Input: part model. Units: mm. Frame: model coordinates. Face numbers are marked on the shaded views. A direction names the side the tool comes from. Round coordinates to 2 decimals unless told otherwise and drop trailing zeros. Order: outer loops, then holes, each group sorted by start corner. A loop starts at its lowest first (then second) coordinate and runs counter-clockwise, first axis right, second up. Notation, with made-up numbers: (0.5, 73.5) -> (10.5, 73.5) arc R8 cw to (10.5, 87.5) -> close; hole circle Ø9 at (84.25, -28). An arc over 180 degrees is marked (long way). Use a Markdown table: item, result.
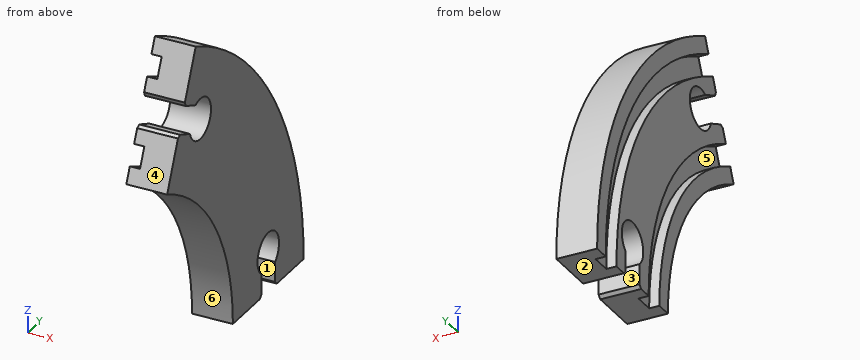
from build123d import *

# Parameters (mm, degrees)
F4_DEPTH = 12.7
F5_SIZE  = 1.016


with BuildPart() as f2:
    # F2: sweep along a path in F1
    with BuildLine(Plane.YZ) as f2_path:
        ThreePointArc((0, 0), (-13.9895526568, 47.0829736144), (-51.4187773904, 78.8881166537))
    # F0 (on Top) → F2 (sweep)
    with BuildSketch(Plane.XY):
        Polygon((-2.9826171882, -15.875), (-2.9826171882, -20.955), (9.7173828118, -20.955), (9.7173828118, 20.955), (-2.9826171882, 20.955), (-2.9826171882, 15.875), (0.1923828118, 15.875), (0.1923828118, 9.525), (-2.9826171882, 9.525), (-2.9826171882, -9.525), (0.1923828118, -9.525), (0.1923828118, -15.875), align=None)
    sweep(path=f2_path.line)

    # F3 (on face) → F4 (cut, through all)
    with BuildSketch(Plane.YZ.offset(9.7173828118)):
        with BuildLine():
            Line((-4.064, 7.3128193311), (-4.064, 0))
            Line((-4.064, 0), (4.064, 0))
            Line((4.064, 0), (4.064, 7.3128193311))
            ThreePointArc((4.064, 7.3128193311), (0, 18.542), (-4.064, 7.3128193311))
        make_face()
        with BuildLine():
            Line((-43.0877289811, 79.6543117793), (-49.7782573242, 82.6062868909))
            Line((-49.7782573242, 82.6062868909), (-53.0592974567, 75.1699464166))
            Line((-53.0592974567, 75.1699464166), (-46.3687691136, 72.217971305))
            ThreePointArc((-46.3687691136, 72.217971305), (-34.4546256835, 71.4032438515), (-43.0877289811, 79.6543117793))
        make_face()
    extrude(amount=-F4_DEPTH, mode=Mode.SUBTRACT)

    # F5
    f5_edges = [f2.edges().sort_by_distance(p)[0] for p in [
        (3.367383, -53.059297, 75.169946),
        (3.367383, -49.778257, 82.606287),
        (3.367383, 4.064, 0),
        (3.367383, -4.064, 0),
    ]]
    chamfer(f5_edges, length=F5_SIZE)


solid = f2.part
1) Pull-direction query (Y, two-part tool) for the marked faces 1, 2, 3 and 4; classes: +Y half, -Y half, draft (parallel to the pull), parting line (faces both ways), or undercut.
Results found:
| item | result |
|---|---|
| face 1 | undercut |
| face 2 | draft |
| face 3 | undercut |
| face 4 | -Y half |
2) Cut plane C-C on y = 0. Return loops of the section in (x, z).
Results found:
| item | result |
|---|---|
| outline | (-2.98, 18.54) -> (9.72, 18.54) -> (9.72, 63.66) -> (-2.98, 63.66) -> (-2.98, 54.68) -> (0.19, 54.68) -> (0.19, 41.63) -> (-2.98, 41.63) -> close |
3) Line query: L1, parallel to Y at x = -0.75, z = 18; L2, parallel to Y at x = -1.5, z = 40; L3, parallel to Y at x = -0.25, z = 69.5. Output: solid intervals per line, ascending. Write a range as [from, to].
Results found:
| item | result |
|---|---|
| L1 | y = [-23.49, -18.22], [-11.67, -2.57], [2.57, 7.82], [14.28, 19.43] |
| L2 | y = [-34.65, -28.35], [-20.78, 0.77], [7.71, 13.21] |
| L3 | y = [-53.78, -44.78], [-35.75, -20.36], [-11.43, -4.63] |
4) Set-up query: the marked faces 5 and 6. Return all of +Z, -Z, +X, -X, +Y, -Y with unobstructed straight access to the full face (end or side cutting, diameter ignored); none if empty.
Results found:
| item | result |
|---|---|
| face 5 | -X |
| face 6 | -Z, +X, -X, -Y |
5) Cut plane A-A on x = 6.5. Return loops of the section in (y, z) (3 decimals), and give its area (3 significant figures).
Results found:
| item | result |
|---|---|
| outline | (-59.878, 59.716) arc R65.271 cw to (-20.955, 0) -> (-5.08, 0) -> (-4.064, 1.016) -> (-4.064, 7.313) arc R6.35 cw (long way) to (4.064, 7.313) -> (4.064, 1.016) -> (5.08, 0) -> (20.955, 0) arc R107.181 ccw to (-42.96, 98.06) -> (-49.368, 83.536) -> (-48.849, 82.196) -> (-43.088, 79.654) arc R6.35 cw (long way) to (-46.369, 72.218) -> (-52.13, 74.76) -> (-53.469, 74.24) -> close |
| area | 3,820 mm² |
6) Pin query (flat end, axial travel): pin 1 Ø4 at (x, y) = (3.5, 10.5) entering from +Z; pin 2 Ø4 at (x, y) = (1, 11.5) entering from +Z; pin 3 Ø5 at (x, z) = (7.5, 69) entering from -Y; pin 4 Ø11.5 at (y, z) = (0, 12.192) entering from +X. Return the tip coordinate at first contact, or that it passes through.
Results found:
| item | result |
|---|---|
| pin 1 | stops at z = 50.15 |
| pin 2 | stops at z = 48.21 |
| pin 3 | stops at y = -56.88 |
| pin 4 | passes through |
7) Cut plane D-D on y = -26.5. Return loops of the section in (x, z), and give its area (3 significant figures).
Results found:
| item | result |
|---|---|
| outline | (-2.98, 26.33) -> (9.72, 26.33) -> (9.72, 89) -> (-2.98, 89) -> (-2.98, 82.81) -> (0.19, 82.81) -> (0.19, 74.84) -> (-2.98, 74.84) -> (-2.98, 48.12) -> (0.19, 48.12) -> (0.19, 37.18) -> (-2.98, 37.18) -> close |
| area | 736 mm² |
8) Cut plane B-B on z = 14.5. Return loops of the section in (x, y), and give its area (3 significant figures).
Results found:
| item | result |
|---|---|
| outline | (-2.98, -22.59) -> (9.72, -22.59) -> (9.72, -5.92) -> (-2.98, -5.92) -> (-2.98, -10.91) -> (0.19, -10.91) -> (0.19, -17.39) -> (-2.98, -17.39) -> close; (-2.98, 5.92) -> (9.72, 5.92) -> (9.72, 19.97) -> (-2.98, 19.97) -> (-2.98, 14.84) -> (0.19, 14.84) -> (0.19, 8.42) -> (-2.98, 8.42) -> close |
| area | 349 mm² |
